For this review, use the dimensioned drawing (mm, ordinates from the lowest corner) and the shaded views. Coordinates: 2 decimals unless noted, no trailing zeros. Write each loop counter-clockwise with the first axis right and the second up, starting at its lowest first coordinate (ties: lowest second). Pieces come first, ordered by that corner, then holes. Notation, with made-up numbers: (27.5, 10) - (42.5, 10) arc R16 ccw to (42.5, 25) - close; hole circle Ø2 at (-26.5, 2). An arc over 180 degrees is marked (long way). Answer as a JSON object with one key per item and string values.
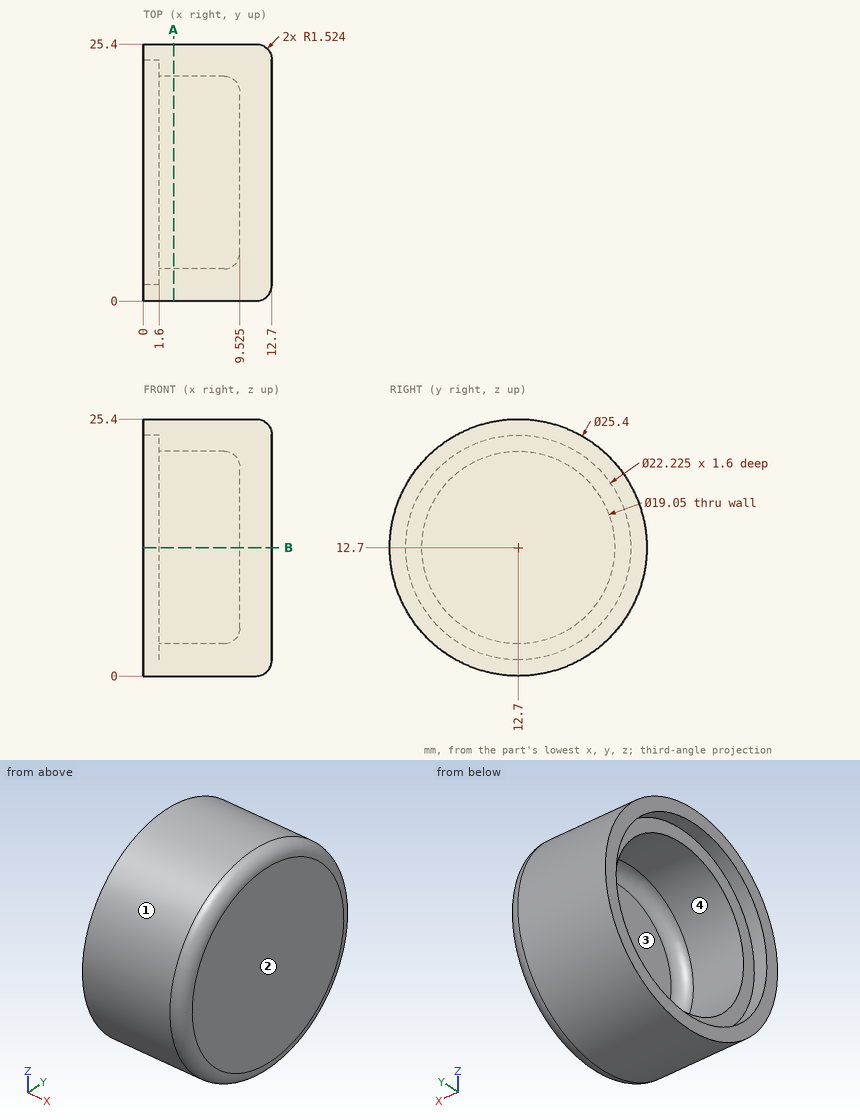
(1) The part is to be moulded in two halves that separate along Z. For the marked faces 1, 2, 3 and 4, say which applies: pulls with the +Z half, pulls with the -Z half, needs draft (parallel to the pull), parting line crosses it, or undercut.
Solved:
{"face 1": "parting line crosses it", "face 2": "needs draft", "face 3": "undercut", "face 4": "undercut"}
(2) For pin 1 (4 mm diameter, centred on x = 6.5, y = 17, fed in from -Z); pin 2 (12 mm diameter, centred on y = 9.5, z = 16.5, fed in from -X); pin 3 (1 mm diameter, centred on x = 6, y = 18.5, fed in from -Z), all flat-tipped, find the tip position at first contact; note any pin that passes through.
Solved:
{"pin 1": "stops at z = 0.21", "pin 2": "stops at x = 1.6", "pin 3": "stops at z = 1.16"}
(3) Take a section at A-A, the plane x = 3. Write out the cut boundary in (y, z) (3 decimals).
Solved:
{"outline": "circle Ø25.4 at (12.7, 12.7); hole circle Ø19.05 at (12.7, 12.7)"}
(4) To check wall thickness, follow line 1 (Y direction, x = 0.95, z = 12.7); line 2 (Y direction, x = 4.75, z = 12.7) (3 decimals); line 3 (X direction, y = 6.25, z = 17) (3 decimals). State the ranges of each line that lie inside material, in increasing order. Write a range as from..to.
Solved:
{"line 1": "y = 0..1.59, 23.81..25.4", "line 2": "y = 0..3.175, 22.225..25.4", "line 3": "x = 9.525..12.7"}
(5) Take a section at B-B, the plane z = 12.7. Write out the cut boundary in (x, y) (1 decimal).
Solved:
{"outline": "(0, 0) - (11.2, 0) arc R1.5 ccw to (12.7, 1.5) - (12.7, 23.9) arc R1.5 ccw to (11.2, 25.4) - (0, 25.4) - (0, 23.8) - (1.6, 23.8) - (1.6, 22.2) - (8, 22.2) arc R1.5 cw to (9.5, 20.7) - (9.5, 4.7) arc R1.5 cw to (8, 3.2) - (1.6, 3.2) - (1.6, 1.6) - (0, 1.6) - close"}
